```python
from build123d import *
from build123d.topology import SkipClean

# Parameters (mm, degrees)
BOSS_EXTRUDE1_DEPTH = 6.35
SKETCH3_R           = 3.5
CUT_EXTRUDE1_DEPTH  = 4
FILLET1_R           = 1
SKETCH4_R           = 12.5
BOSS_EXTRUDE2_DEPTH = 6.35
CUT_EXTRUDE2_DEPTH  = 13.7
FILLET2_R           = 1
FILLET3_R           = 1.5875
SKETCH9_R           = 3.5
CUT_EXTRUDE3_DEPTH  = 2.2


with BuildPart() as part:
    # Sketch2 → Boss-Extrude1 (new body)
    with BuildSketch(Plane(origin=(0, 0, 0), x_dir=(0, 0, -1), z_dir=(1, 0, 0))):
        with BuildLine():
            Line((-12.449272067, -1.125), (-7.967534123, -50.72))
            ThreePointArc((-7.967534123, -50.72), (0, -58), (7.967534123, -50.72))
            Line((7.967534123, -50.72), (12.449272067, -1.125))
            ThreePointArc((12.449272067, -1.125), (12.5, 0), (12.449272067, 1.125))
            Line((12.449272067, 1.125), (7.967534123, 50.72))
            ThreePointArc((7.967534123, 50.72), (0, 58), (-7.967534123, 50.72))
            Line((-7.967534123, 50.72), (-12.449272067, 1.125))
            ThreePointArc((-12.449272067, 1.125), (-12.5, 0), (-12.449272067, -1.125))
        make_face()
    extrude(amount=-BOSS_EXTRUDE1_DEPTH)

    # Sketch3 → Cut-Extrude1 (cut)
    with BuildSketch(Plane.ZY.offset(6.35)):
        with BuildLine():
            Line((-4.118569102, 56.858380899), (1.62233922, 54.993046711))
            ThreePointArc((1.62233922, 54.993046711), (5.25, 50), (1.62233922, 45.006953289))
            Line((1.62233922, 45.006953289), (-8.789515625, 41.623936576))
            Line((-8.789515625, 41.623936576), (-7.967534123, 50.72))
            ThreePointArc((-7.967534123, 50.72), (-6.777787456, 54.249893786), (-4.118569102, 56.858380899))
        make_face()
        with Locations((0, 50)):
            Circle(SKETCH3_R, mode=Mode.SUBTRACT)
    cut_extrude1 = extrude(amount=-CUT_EXTRUDE1_DEPTH, mode=Mode.SUBTRACT)

    # Fillet1
    fillet1_edges = [part.edges().sort_by_distance(p)[0] for p in [
        (-4.35, 56.858380899, -4.118569102),
        (-4.35, 41.623936576, -8.789515625),
    ]]
    fillet(fillet1_edges, radius=FILLET1_R)

    # Mirror1: Cut-Extrude1 across plane
    add(cut_extrude1.mirror(Plane.ZX), mode=Mode.SUBTRACT)

    # Sketch4 → Boss-Extrude2 (add)
    with SkipClean():  # keep this step's faces unmerged: merging them makes the solid invalid here
        with BuildSketch(Plane.ZY.offset(6.35)):
            with Locations(Location((0, 0, 0), (0, 0, 174.836392909))):  # turned: the seam where the file's is
                Circle(SKETCH4_R)
        extrude(amount=BOSS_EXTRUDE2_DEPTH)

    # Sketch5 → Cut-Extrude2 (cut, through all)
    with SkipClean():  # keep this step's faces unmerged: merging them makes the solid invalid here
        with BuildSketch(Plane.ZY.offset(12.7)):
            with BuildLine():
                Line((-3.2258, 5.484356448), (-3.2258, -5.484356448))
                ThreePointArc((-3.2258, -5.484356448), (0, -6.3627), (3.2258, -5.484356448))
                Line((3.2258, -5.484356448), (3.2258, 5.484356448))
                ThreePointArc((3.2258, 5.484356448), (0, 6.3627), (-3.2258, 5.484356448))
            make_face()
        extrude(amount=-CUT_EXTRUDE2_DEPTH, mode=Mode.SUBTRACT)

    # Fillet2
    fillet2_edges = [part.edges().sort_by_distance(p)[0] for p in [
        (-4.35, -56.858380899, -4.118569102),
        (-4.35, -41.623936576, -8.789515625),
    ]]
    fillet(fillet2_edges, radius=FILLET2_R)

    # Fillet3
    fillet3_edges = [part.edges().sort_by_distance(p)[0] for p in [
        (-6.35, 5.484356448, -3.2258),
        (-6.35, 5.484356448, 3.2258),
        (-6.35, -5.484356448, 3.2258),
        (-6.35, -5.484356448, -3.2258),
    ]]
    fillet(fillet3_edges, radius=FILLET3_R)

    # Sketch9 → Cut-Extrude3 (cut)
    with SkipClean():  # keep this step's faces unmerged: merging them makes the solid invalid here
        with BuildSketch(Plane.ZY.offset(6.35)):
            with Locations((0, 50)):
                Circle(SKETCH9_R)
        cut_extrude3 = extrude(amount=-CUT_EXTRUDE3_DEPTH, mode=Mode.SUBTRACT)

    # Sketch7 → #8-32 Tapped Hole1 (revolve, cut)
    with SkipClean():  # keep this step's faces unmerged: merging them makes the solid invalid here
        with BuildSketch(Plane(origin=(-6.35, 50, 0), x_dir=(0, 0, 1), z_dir=(0, 1, 0))):
            Polygon((0, 0), (0, 13.327806461), (1.7272, 12.29), (1.7272, 0), align=None)
        f_8_32_tapped_hole1 = revolve(axis=Axis((-12.7, 50, 0), (1, 0, 0)), mode=Mode.SUBTRACT)

    # Mirror2: Cut-Extrude3, #8-32 Tapped Hole1 across plane
    with SkipClean():  # keep this step's faces unmerged: merging them makes the solid invalid here
        add(cut_extrude3.mirror(Plane.ZX), mode=Mode.SUBTRACT)
        add(f_8_32_tapped_hole1.mirror(Plane.ZX), mode=Mode.SUBTRACT)


solid = part.part
```
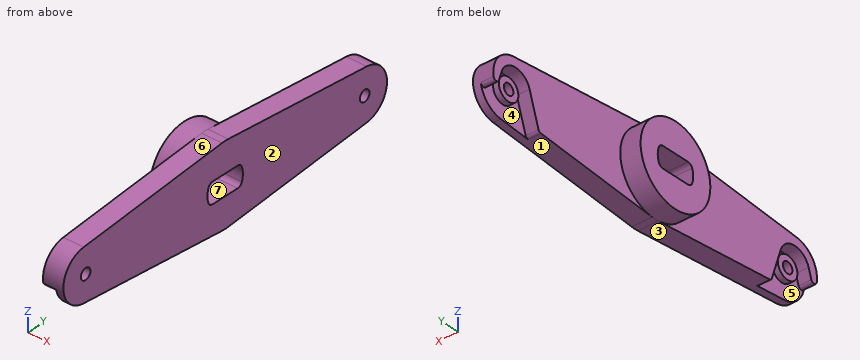
Geometry check sheet. Reference: the model listing, model coordinates, mm. Face numbers are marked on the shaded views. A direction names the side the tool comes from. Coordinates: 2 decimals unless noted, no trailing zeros. Order: outer loops, then holes, each group sorted by start corner. A loop starts at its lowest first (then second) coordinate and runs counter-clockwise, first axis right, second up.
Q1. Tool access check on the marked faces 5, 6 and 7. Record the directions out of +Z, -Z, +X, -X, +Y, -Y that give a thin tool (end or side, any length) a straight path to the whole face; none if there is none.
Reply:
face 5: -X
face 6: +Z, +X, -X, -Y
face 7: +X, -X
Q2. Sectioned sample at C-C on z = -5.5. Record the cut outline in (x, y).
Reply:
outline: (-12.7, -11.22) - (-6.35, -11.22) - (-6.35, -42.69) - (-2.35, -42.69) - (-2.35, -55.81) - (0, -55.81) - (0, 55.81) - (-2.35, 55.81) - (-2.35, 42.69) - (-6.35, 42.69) - (-6.35, 11.22) - (-12.7, 11.22) - close
Q3. Sectioned sample at A-A on x = -7.5. Record the cut outline in (y, z) (1 decimal), and give its area (3 significant figures).
Reply:
outline: circle Ø25 at (0, 0); hole (-6, -2.2) arc R1.6 ccw to (-4.5, -3.2) - (4.5, -3.2) arc R1.6 ccw to (6, -2.2) arc R6.4 ccw to (6, 2.2) arc R1.6 ccw to (4.5, 3.2) - (-4.5, 3.2) arc R1.6 ccw to (-6, 2.2) arc R6.4 ccw to start
area: 413 mm2
Q4. Sectioned sample at D-D on z = 0. Give the number of separate pieces and of enclosed holes in the cut face, and give its area (3 significant figures).
Reply:
separate pieces: 4
enclosed holes: 0
area: 642 mm2
Q5. Sectioned sample at B-B on y = 0. Record the cut outline in (x, z), and give its area (3 significant figures).
Reply:
outline: (-12.7, -12.5) - (0, -12.5) - (0, -3.23) - (-12.7, -3.23) - close; (-12.7, 3.23) - (0, 3.23) - (0, 12.5) - (-12.7, 12.5) - close
area: 236 mm2
Q6. Depth check by flat-ended pin: pin 1 Ø2.5 at (x, y) = (-5.5, -1) entering from -Z; pin 2 Ø3.5 at (y, z) = (-51, 1) entering from -X; pin 3 Ø7 at (y, z) = (48, 0) entering from -X; pin 4 Ø5 at (x, y) = (-7.5, 19.5) entering from -Z. Enter the tip coordinate at first touch or a pass-through.
Reply:
pin 1: stops at z = -12.5
pin 2: stops at x = -4.15
pin 3: stops at x = -6.35
pin 4: stops at z = -10.99
Q7. Draft check along Y on the marked faces 1, 2, 3 and 4. Enter one of: released by +Y, released by -Y, zero draft, split by the parting line, or undercut.
Reply:
face 1: released by +Y
face 2: zero draft
face 3: released by -Y
face 4: undercut
Q8. Thickness scan on probe 1 along Y at (x, z) = (-0.9, 0); probe 2 along X at (y, z) = (-26, -7); probe 3 along Z at (x, y) = (-4.5, 3.5). Record the ranges inside material, lowest first.
Reply:
probe 1: y = -58 to -51.73, -48.27 to -6.36, 6.36 to 48.27, 51.73 to 58
probe 2: x = -6.35 to 0
probe 3: z = -12.23 to -3.23, 3.23 to 12.23
